Source: CAD feature listing. Evaluate the final solid. Frame: model axes, mm. A direction names the side the tool comes from. Give positions to 0.01 mm unless a question says otherwise; leave off trailing zeros. Write each loop counter-clockwise with the first axis right and the second up, starting at its lowest first coordinate (ties: lowest second). Pieces come first, ordered by that corner, then holes. Notation, with made-up numbers: M 50.5,35.5 L 90.5,35.5 A21 ccw 90.5,47.5 Z; hole C 12,-24.75 d5. An arc over 180 degrees is marked long. Use CSV: the item, a comma, the result in double quotes. Start each with the question number.
Autodesk Inventor part; units mm, degrees
ref_plane "YZ Plane" through (0, 0, 0) normal (1, 0, 0) x (0, 1, 0)
ref_plane "XZ Plane" through (0, 0, 0) normal (0, 1, 0) x (-1, 0, 0)
ref_plane "XY Plane" through (0, 0, 0) normal (0, 0, 1) x (1, 0, 0)
sketch "Sketch1" plane through (0, 0, 0) normal (0, 0, 1) x (1, 0, 0)
  circle A0 centre (0, 0) radius 4.9301
  circle A1 centre (0, 0) radius 8.5
  dimension "d0" = 9.8602
  dimension "d1" = 17
extrude "Extrusion1" add sketch "Sketch1" along normal blind 9
sketch "Sketch2" plane through (0, 0, 9) normal (0, 0, 1) x (1, 0, 0)
  line L0 (-7.5, 7.5) -> (7.5, 7.5)
  line L1 (7.5, 7.5) -> (7.5, -7.5)
  line L2 (7.5, -7.5) -> (-7.5, -7.5)
  line L3 (-7.5, -7.5) -> (-7.5, 7.5)
  line L4 (0, 0) -> (0, 8.3867)
  line L5 (0, 0) -> (9.7878, 0)
  circle A0 centre (0, 0) radius 10.6066
  point P0 (0, 7.5)
  point P1 (7.5, 0)
  dimension "d4" = 15
extrude "Extrusion2" cut sketch "Sketch2" against normal blind 3 contours A0 L0 | L3 A0 | L2 A0 | A0 L1
properties part number "TuercaD_eje" material "Steel"
Item 1: Material intervals for probe 1 along Y at (x, z) = (0, 4.75); probe 2 along Y at (x, z) = (0, 6.5); probe 3 along X at (y, z) = (0.75, 4), sorted ascending.
Item 2: Pull-direction query (X, two-part tool) for faces 6 (the cylindrical face through (4.702, -1.481, 4.437)), 7 (the cylindrical face through (-6.265, -5.745, 3.437)), 8 (the flat face through (0, 7.5, 8)); classes: released by +X, released by -X, zero draft, split by the parting line, or undercut.
Item 3: Section D-D (x = -4.5). Return the cut outline in (y, z), plus the area to 3 significant figures.
Item 4: Contact query for flat-ended pins moving along their axis: pin 1 Ø1.5 at (y, z) = (-5, 4.5) entering from +X; pin 2 Ø1.5 at (x, z) = (-2, 2.5) entering from -Y; pin 3 Ø5 at (x, z) = (-4.5, 5) entering from -Y. Output: stop coordinate, or through.
Item 5: Section A-A (y = 0). Return the cut outline in (x, z), plus the area to 3 significant figures.
Item 6: Set-up query: faces 1 (the flat face through (0, 8, 6)), 2 (the flat face through (0, -8, 6)), 3 (the flat face through (-0.1, 5.1, 9)), 4 (the flat face through (-8, 0, 6)), 5 (the flat face through (8, 0, 6)). Return all of +Z, -Z, +X, -X, +Y, -Y with unobstructed straight access to the full face (end or side cutting, diameter ignored); none if empty.
Item 7: Section C-C (z = 7). Return the cut outline in (x, y).
Output values:
1,probe 1,"y = -8.5 to -4.93, 4.93 to 8.5"
1,probe 2,"y = -7.5 to -4.93, 4.93 to 7.5"
1,probe 3,"x = -8.47 to -4.87, 4.87 to 8.47"
2,face 6,"undercut"
2,face 7,"split by the parting line"
2,face 8,"zero draft"
3,outline,"M -7.21,0 L -2.01,0 L -2.01,9 L -7.21,9 Z; M 2.01,0 L 7.21,0 L 7.21,9 L 2.01,9 Z"
3,area,"93.5 mm2"
4,pin 1,"stops at x = 7.36"
4,pin 2,"stops at y = -8.41"
4,pin 3,"stops at y = -8.26"
5,outline,"M -8.5,0 L -4.93,0 L -4.93,9 L -7.5,9 L -7.5,6 L -8.5,6 Z; M 4.93,0 L 8.5,0 L 8.5,6 L 7.5,6 L 7.5,9 L 4.93,9 Z"
5,area,"58.3 mm2"
6,face 1,"+Z, +X, -X, +Y"
6,face 2,"+Z, +X, -X, -Y"
6,face 3,"+Z, +X, -X, +Y, -Y"
6,face 4,"+Z, -X, +Y, -Y"
6,face 5,"+Z, +X, +Y, -Y"
7,outline,"M -7.5,-4 A8.5 ccw -4,-7.5 L 4,-7.5 A8.5 ccw 7.5,-4 L 7.5,4 A8.5 ccw 4,7.5 L -4,7.5 A8.5 ccw -7.5,4 Z; hole C 0,0 d9.86"
